from build123d import *

# Parameters (mm, degrees)
BOSS_EXTRUDE1_DEPTH                = 38
F_3_0_3_DIAMETER_HOLE1_D           = 3
F_3_0_3_DIAMETER_HOLE1_CSINK_D     = 3.05
F_3_0_3_DIAMETER_HOLE1_CSINK_ANGLE = 90
SKETCH6_W                          = 4
SKETCH6_H                          = 4
BOSS_EXTRUDE2_DEPTH                = 24
FILLET2_R                          = 7
FILLET3_START                      = 7.489649075
FILLET3_DEPTH                      = 4
FILLET3_START_2                    = 26.489649075
FILLET3_2_DEPTH                    = 4
FILLET3_START_3                    = 1.165093755
FILLET3_3_DEPTH                    = 6.32455532
FILLET3_START_4                    = 30.489649075
FILLET3_4_DEPTH                    = 6.324555321
FILLET3_START_5                    = -11
FILLET3_5_DEPTH                    = 7
SKETCH7_W                          = 15
SKETCH7_H                          = 4
BOSS_EXTRUDE3_DEPTH                = 4
FILLET4_R                          = 7
FILLET5_R                          = 3


with BuildPart() as part:
    # Sketch1 → Boss-Extrude1 (new body)
    with BuildSketch(Plane(origin=(0, 0, 0), x_dir=(0, 0, -1), z_dir=(1, 0, 0))):
        Polygon((-20, 15), (20, 15), (100, -15), (20, -15), (-20, -15), align=None)
    extrude(amount=BOSS_EXTRUDE1_DEPTH)

    # Ø3.0 (3) Diameter Hole1 (through all)
    with Locations(Plane.ZY):
        with Locations((17.5, 12.5), (-17.5, 12.5), (-17.5, -12.5), (17.5, -12.5)):
            CounterSinkHole(F_3_0_3_DIAMETER_HOLE1_D / 2, F_3_0_3_DIAMETER_HOLE1_CSINK_D / 2, counter_sink_angle=F_3_0_3_DIAMETER_HOLE1_CSINK_ANGLE)

    # Sketch6 → Boss-Extrude2 (add)
    with BuildSketch(Plane.XY.offset(20)):
        with Locations((9.489649075, 17)):
            Rectangle(SKETCH6_W, SKETCH6_H)
        with Locations((28.489649075, 17)):
            Rectangle(SKETCH6_W, SKETCH6_H)
    extrude(amount=-BOSS_EXTRUDE2_DEPTH)

    # Fillet2
    # the kernel refuses this fillet: 7 mm, written as the material it adds along each edge
    with BuildSketch(Plane(origin=(30.489649075, 15, 20), x_dir=(1, 0, 0), z_dir=(0, 0, -1))) as fillet2_piece_1:
        with BuildLine():
            CenterArc((6.32455532, -7), FILLET2_R, 90, 64.623066475)
            Line((0, -4), (-0.126491106, -3.94))
            ThreePointArc((-0.126491106, -3.94), (-0.14, -2), (-0.14, 0))
            Line((-0.14, 0), (0, 0.14))
            Line((0, 0.14), (6.32455532, 0.14))
            Line((6.32455532, 0.14), (6.32455532, 0))
        make_face()
    extrude(amount=24)
    with BuildSketch(Plane(origin=(7.489649075, 15, 20), x_dir=(-1, 0, 0), z_dir=(0, 0, -1))) as fillet2_piece_2:
        with BuildLine():
            CenterArc((6.32455532, 7), FILLET2_R, 205.376933525, 64.623066475)
            Line((0, 4), (-0.126491106, 3.94))
            ThreePointArc((-0.126491106, 3.94), (-0.14, 2), (-0.14, 0))
            Line((-0.14, 0), (0, -0.14))
            Line((0, -0.14), (6.32455532, -0.14))
            Line((6.32455532, -0.14), (6.32455532, 0))
        make_face()
    extrude(amount=24)

    # Fillet3: read off the stored shape, not the designer's step
    # Fillet3 outline → Fillet3 (add)
    with BuildSketch(Plane.YZ.offset(FILLET3_START)):
        with BuildLine():
            Line((15, -4), (15, -10.32455532))
            ThreePointArc((15, -10.32455532), (16.083920217, -6.582897934), (19, -4))
            Line((19, -4), (15, -4))
        make_face()
    extrude(amount=FILLET3_DEPTH)

    # Fillet3 2 outline → Fillet3 2 (add)
    with BuildSketch(Plane.YZ.offset(FILLET3_START_2)):
        with BuildLine():
            Line((15, -4), (15, -10.32455532))
            ThreePointArc((15, -10.32455532), (16.083920217, -6.582897934), (19, -4))
            Line((19, -4), (15, -4))
        make_face()
    extrude(amount=FILLET3_2_DEPTH)

    # Fillet3 3 outline → Fillet3 3 (add)
    with BuildSketch(Plane.YZ.offset(FILLET3_START_3)):
        with BuildLine():
            Line((15, -4), (15, -10.32455532))
            ThreePointArc((15, -10.32455532), (16.083920217, -6.582897934), (19, -4))
            Line((19, -4), (15, -4))
        make_face()
    extrude(amount=FILLET3_3_DEPTH)

    # Fillet3 4 outline → Fillet3 4 (add)
    with BuildSketch(Plane.YZ.offset(FILLET3_START_4)):
        with BuildLine():
            Line((15, -4), (15, -10.32455532))
            ThreePointArc((15, -10.32455532), (16.083920217, -6.582897934), (19, -4))
            Line((19, -4), (15, -4))
        make_face()
    extrude(amount=FILLET3_4_DEPTH)

    # Fillet3 5 outline → Fillet3 5 (cut)
    with BuildSketch(Plane.XY.offset(FILLET3_START_5)):
        with BuildLine():
            Line((30.015307426, 20), (30.489649075, 19))
            ThreePointArc((30.489649075, 19), (33.072547009, 16.083920217), (36.814204396, 15))
            Line((36.814204396, 15), (36.814204396, 20))
            Line((36.814204396, 20), (30.015307426, 20))
        make_face()
        with BuildLine():
            Line((7.489649075, 19), (7.963990724, 20))
            Line((7.963990724, 20), (1.165093755, 20))
            Line((1.165093755, 20), (1.165093755, 15))
            ThreePointArc((1.165093755, 15), (4.906751142, 16.083920217), (7.489649075, 19))
        make_face()
    extrude(amount=FILLET3_5_DEPTH, mode=Mode.SUBTRACT)

    # Sketch7 → Boss-Extrude3 (add)
    with BuildSketch(Plane(origin=(0, 15, 0), x_dir=(1, 0, 0), z_dir=(0, 1, 0))):
        with Locations((18.989649075, 2)):
            Rectangle(SKETCH7_W, SKETCH7_H)
    extrude(amount=BOSS_EXTRUDE3_DEPTH)

    # Fillet4
    # the kernel refuses this fillet: 7 mm, written as the material it adds along each edge
    with BuildSketch(Plane(origin=(11.489649075, 15, -4), x_dir=(0, 0, -1), z_dir=(1, 0, 0))) as fillet4_piece_1:
        with BuildLine():
            CenterArc((6.32455532, 7), FILLET4_R, 205.376933525, 64.623066475)
            Line((0, 4), (-0.126491106, 3.94))
            ThreePointArc((-0.126491106, 3.94), (-0.14, 2), (-0.14, 0))
            Line((-0.14, 0), (0, -0.14))
            Line((0, -0.14), (6.32455532, -0.14))
            Line((6.32455532, -0.14), (6.32455532, 0))
        make_face()
    extrude(amount=15)

    # Fillet5
    # the kernel refuses this fillet: 3 mm, written as the material it takes off along each edge
    with BuildSketch(Plane(origin=(30.489649075, 19, 24.188611699), x_dir=(-1, 0, 0), z_dir=(0, 0, -1))) as fillet5_piece_1:
        with BuildLine():
            CenterArc((1.67544468, -3), FILLET5_R, 90, 53.130102354)
            ThreePointArc((-0.72455532, -1.2), (-0.332163903, -0.618182569), (0, 0))
            Line((0, 0), (1.67544468, 0))
        make_face()
    extrude(amount=32.377223398, mode=Mode.SUBTRACT)
    with BuildSketch(Plane(origin=(34.678260774, 19, -4), x_dir=(0, 0, 1), z_dir=(-1, 0, 0)), Plane(origin=(11.489649075, 19, -4), x_dir=(0, 0, 1), z_dir=(-1, 0, 0))) as fillet5_piece_2:
        with BuildLine():
            CenterArc((1.675444679, -3), FILLET5_R, 90, 53.130102349)
            ThreePointArc((-0.72455532, -1.2), (-0.332163903, -0.618182569), (0, 0))
            Line((0, 0), (1.675444679, 0))
        make_face()
    extrude(amount=8.188611699, mode=Mode.SUBTRACT)
    with BuildSketch(Plane(origin=(11.489649075, 19, -4), x_dir=(0, -0.8560559167430235, -0.5168832241515113), z_dir=(1, 0, 0))) as fillet5_piece_3:
        with BuildLine():
            CenterArc((1.702158502, -2.984924004), FILLET5_R, 95.74648206, 53.130102354)
            Line((-0.866009248, -1.434274331), (0, 0))
            ThreePointArc((0, 0), (0.700888795, -0.035177325), (1.40177759, 0))
        make_face()
    extrude(amount=15, mode=Mode.SUBTRACT)
    with BuildSketch(Plane(origin=(7.489649075, 19, 24.188611699), x_dir=(1, 0, 0), z_dir=(0, 0, -1))) as fillet5_piece_4:
        with BuildLine():
            CenterArc((1.67544468, 3), FILLET5_R, 216.869897646, 53.130102354)
            ThreePointArc((-0.72455532, 1.2), (-0.332163903, 0.618182569), (0, 0))
            Line((0, 0), (1.67544468, 0))
        make_face()
    extrude(amount=32.377223398, mode=Mode.SUBTRACT)


solid = part.part
The listing builds one solid part. Answer for the finished solid, in the listing's coordinates (mm). A direction names the side the tool comes from. Coordinates: 2 decimals unless noted, no trailing zeros. Order: outer loops, then holes, each group sorted by start corner. A loop starts at its lowest first (then second) coordinate and runs counter-clockwise, first axis right, second up. Notation, with made-up numbers: (-6.5, 43) -> (0.5, 43) arc R24 cw to (0.5, 79) -> close; hole circle Ø11 at (-19.75, 23.25). An arc over 180 degrees is marked (long way). Answer in a Markdown table with one row per item. Add a question column.
Item 1: Which of the six approach directions +Z, -Z, +X, -X, +Y, -Y give full straight-line access (tool end or side, diameter ignored) to faces 1 (the face through (19.28, -12.43, -16)), 2 (the face through (19, 17, 0))?
Item 2: Find the intervals of material crossed by L1, parallel to Y at x = 19.5, z = 17.5; L2, parallel to Y at x = 24, z = 17; L3, parallel to Y at x = 19, z = -42, in increasing order. Write a range as from..to.
Item 3: Determine the mould class of faces 3 (the face through (18.73, 0.21, -59.44)), 4 (the face through (19.28, 12.57, 19)), 5 (the face through (30.14, 18.69, 7.81)) for opening direction Z: +Z half, -Z half, draft (parallel to the pull), parting line (faces both ways), or undercut.
Item 4: Find section A-A (z = 17.5). Write down the section's boundary in (x, y) (3 decimals), then the cut area to 3 significant figures.
Item 5: Find section C-C (y = -12.5). Write down the section's boundary in (x, z) (3 decimals), then the cut area to 3 significant figures.
Item 6: Find section B-B (x = 13). Write down the section's boundary in (y, z).
Item 7: Each of these flat-tipped pins is pushed along its axis until it touches: P1, Ø3.5, axis at y = -12.5, z = -17.5, coming from the -X side; P2, Ø7.5, axis at x = 19.5, z = 13.5, coming from the +Y side; P3, Ø2.5, axis at y = 12.5, z = 17.5, coming from the +X side. Where does it stop, or does it pass through?
Item 8: Find section D-D (z = -24). Write down the section's boundary in (x, y).
Result set:
| question | item | result |
|---|---|---|
| 1 | face 1 | +X, -X |
| 1 | face 2 | +Z, +Y |
| 2 | L1 | y = -15..-14, -11..11, 14..15 |
| 2 | L2 | y = -15..-13.91, -11.09..11.09, 13.91..15 |
| 2 | L3 | y = -15..6.75 |
| 3 | face 3 | -Z half |
| 3 | face 4 | undercut |
| 3 | face 5 | draft |
| 4 | outline | (0, -15) -> (38, -15) -> (38, -14) -> (0.025, -14) -> (0, -14.025) -> close; (0, -10.975) -> (0.025, -11) -> (38, -11) -> (38, 11) -> (0.025, 11) -> (0, 10.975) -> close; (0, 14.025) -> (0.025, 14) -> (38, 14) -> (38, 15) -> (36.814, 15) arc R7 cw to (31.214, 17.8) arc R3 ccw to (28.814, 19) -> (26.49, 19) -> (26.49, 15) -> (11.49, 15) -> (11.49, 19) -> (9.165, 19) arc R3 ccw to (6.765, 17.8) arc R7 cw to (1.165, 15) -> (0, 15) -> close |
| 4 | area | 958 mm² |
| 5 | outline | (0, -93.333) -> (38, -93.333) -> (38, -19) -> (0.025, -19) -> (0, -19.025) -> close; (0, -15.975) -> (0.025, -16) -> (38, -16) -> (38, 16) -> (0.025, 16) -> (0, 15.975) -> close; (0, 19.025) -> (0.025, 19) -> (38, 19) -> (38, 20) -> (0, 20) -> close |
| 5 | area | 4,080 mm² |
| 6 | outline | (-15, -100) -> (15, -20) -> (15, -10.32) arc R7 cw to (17.8, -4.72) arc R3 ccw to (19, -2.32) -> (19, 0) -> (15, 0) -> (15, 20) -> (-15, 20) -> close; hole circle Ø3 at (-12.5, -17.5); hole circle Ø3 at (-12.5, 17.5); hole circle Ø3 at (12.5, -17.5); hole circle Ø3 at (12.5, 17.5) |
| 7 | P1 | stops at x = 0 |
| 7 | P2 | stops at y = 15 |
| 7 | P3 | passes through |
| 8 | outline | (0, -15) -> (38, -15) -> (38, 13.5) -> (0, 13.5) -> close |
